```python
from build123d import *

# Parameters (mm, degrees)
SKETCH1_R           = 3.25
BOSS_EXTRUDE1_DEPTH = 1.21
SKETCH2_R           = 5.05
BOSS_EXTRUDE2_DEPTH = 8.5
SKETCH3_R           = 2.45
BOSS_EXTRUDE3_DEPTH = 1.9
FILLET1_R           = 1.75
FILLET2_R           = 1.75
SKETCH4_R           = 1.65
CUT_EXTRUDE1_DEPTH  = 14.630740992
SKETCH5_R           = 2.45
CUT_EXTRUDE3_DEPTH  = 8.6


with BuildPart() as part:
    # Sketch1 → Boss-Extrude1 (new body)
    with BuildSketch(Plane(origin=(0, 0, 0), x_dir=(1, 0, 0), z_dir=(0, 1, 0))):
        with Locations(Location((0, 0, 0), (0, 0, 90))):
            Circle(SKETCH1_R)
    extrude(amount=BOSS_EXTRUDE1_DEPTH)

    # Sketch2 → Boss-Extrude2 (add)
    with BuildSketch(Plane(origin=(0, 1.21, 0), x_dir=(1, 0, 0), z_dir=(0, 1, 0))):
        with Locations(Location((0, 0, 0), (0, 0, 270))):
            Circle(SKETCH2_R)
    extrude(amount=BOSS_EXTRUDE2_DEPTH)

    # Sketch3 → Boss-Extrude3 (add)
    with BuildSketch(Plane(origin=(0, 9.71, 0), x_dir=(1, 0, 0), z_dir=(0, 1, 0))):
        with Locations(Location((0, 0, 0), (0, 0, 90))):
            Circle(SKETCH3_R)
    extrude(amount=BOSS_EXTRUDE3_DEPTH)

    # Fillet1
    fillet1_edges = [part.edges().sort_by_distance(p)[0] for p in [
        (0, 9.71, -5.05),
    ]]
    fillet(fillet1_edges, radius=FILLET1_R)

    # Fillet2
    fillet2_edges = [part.edges().sort_by_distance(p)[0] for p in [
        (0, 1.21, -5.05),
    ]]
    fillet(fillet2_edges, radius=FILLET2_R)

    # Sketch4 → Cut-Extrude1 (cut, through all)
    with BuildSketch(Plane(origin=(0, 11.61, 0), x_dir=(1, 0, 0), z_dir=(0, 1, 0))):
        with Locations(Location((0, 0, 0), (0, 0, 270))):
            Circle(SKETCH4_R)
    extrude(amount=-CUT_EXTRUDE1_DEPTH, mode=Mode.SUBTRACT)

    # Sketch5 → Cut-Extrude3 (cut)
    with BuildSketch(Plane.XZ):
        with Locations(Location((0, 0, 0), (0, 0, 270))):
            Circle(SKETCH5_R)
    extrude(amount=-CUT_EXTRUDE3_DEPTH, mode=Mode.SUBTRACT)


solid = part.part
```
Work out the finished part from the listing and answer in its coordinate system (mm). A direction names the side the tool comes from. Round coordinates to 2 decimals unless told otherwise and drop trailing zeros. Loops run counter-clockwise (first coordinate to the right, second up) from the corner with the lowest first, then second, coordinate; pieces in that order, holes last. Notation, with made-up numbers: (59, 12.25) -> (96, 12.25) arc R12 ccw to (96, 30.25) -> close; hole circle Ø11 at (73, 41.25). An arc over 180 degrees is marked (long way). Write each question's results on one line, items separated by ' | '. Start each with the question number.
1. Section D-D (y = 2.5) is taken. Determine the outline of the cut face in (x, z), plus the area to 3 significant figures.
2. Section B-B (x = 0) is taken. Determine the outline of the cut face in (y, z).
3. For a pull along X with two mould halves and no side action, classify faces 4 (the face through (-1, 10.13, -1.31)), 5 (the face through (1.978, 0.597, 2.579)), 6 (the face through (2, 11.61, -1)) as +X half, -X half, draft (parallel to the pull), parting line (faces both ways), or undercut.
4. Given pin 1 Ø3 at (x, z) = (0, 0) entering from +Y; pin 2 Ø1.5 at (y, z) = (6, -3) entering from -X; pin 3 Ø4 at (x, y) = (-3.5, 5) entering from +Z; pin 4 Ø2.5 at (x, z) = (0, -0.5) entering from -Y, each flat-ended and moving along its own axis, determine where each tip first touches the part or whether it passes through.
5. A tool of negligible diameter and unlimited length cuts with its end or side. For faces 1 (the face through (-3.07, 5.42, -4.01)), 2 (the face through (-0.736, 10.647, -2.337)), 3 (the face through (-2, 8.6, -1)), from which of +Z, -Z, +X, -X, +Y, -Y can it reach the whole face along a straight path? Write none if from no direction.
6. Section C-C (y = 4) is taken. Determine the outline of the cut face in (x, z), plus the area to 3 significant figures.
7. Section A-A (z = 0) is taken. Determine the outline of the cut face in (x, y), plus the area to 3 significant figures.
8. Find the intervals of material crossed by probe 1 along X at (y, z) = (6.25, 0); probe 2 along Y at (x, z) = (-0.5, -1.75); probe 3 along X at (y, z) = (10.35, 0), in increasing order. Write a range as from..to.
Evaluation:
1) outline: circle Ø9.98 at (0, 0); hole circle Ø4.9 at (0, 0) | area: 59.3 mm2
2) outline: (0, -3.25) -> (1.21, -3.25) -> (1.21, -3.3) arc R1.75 ccw to (2.96, -5.05) -> (7.96, -5.05) arc R1.75 ccw to (9.71, -3.3) -> (9.71, -2.45) -> (11.61, -2.45) -> (11.61, -1.65) -> (8.6, -1.65) -> (8.6, -2.45) -> (0, -2.45) -> close; (0, 2.45) -> (8.6, 2.45) -> (8.6, 1.65) -> (11.61, 1.65) -> (11.61, 2.45) -> (9.71, 2.45) -> (9.71, 3.3) arc R1.75 ccw to (7.96, 5.05) -> (2.96, 5.05) arc R1.75 ccw to (1.21, 3.3) -> (1.21, 3.25) -> (0, 3.25) -> close
3) face 4: undercut | face 5: parting line | face 6: draft
4) pin 1: passes through | pin 2: stops at x = -4.52 | pin 3: stops at z = 4.82 | pin 4: stops at y = 8.6
5) face 1: +Y, -Y | face 2: +Y | face 3: -Y
6) outline: circle Ø10.1 at (0, 0); hole circle Ø4.9 at (0, 0) | area: 61.3 mm2
7) outline: (-5.05, 2.96) arc R1.75 ccw to (-3.3, 1.21) -> (-3.25, 1.21) -> (-3.25, 0) -> (-2.45, 0) -> (-2.45, 8.6) -> (-1.65, 8.6) -> (-1.65, 11.61) -> (-2.45, 11.61) -> (-2.45, 9.71) -> (-3.3, 9.71) arc R1.75 ccw to (-5.05, 7.96) -> close; (1.65, 8.6) -> (2.45, 8.6) -> (2.45, 0) -> (3.25, 0) -> (3.25, 1.21) -> (3.3, 1.21) arc R1.75 ccw to (5.05, 2.96) -> (5.05, 7.96) arc R1.75 ccw to (3.3, 9.71) -> (2.45, 9.71) -> (2.45, 11.61) -> (1.65, 11.61) -> close | area: 48.3 mm2
8) probe 1: x = -5.05..-2.45, 2.45..5.05 | probe 2: y = 8.6..11.61 | probe 3: x = -2.45..-1.65, 1.65..2.45
